Design review of the part built by this model. Coordinates are the model's own, in mm. Face numbers are marked on the shaded views. A direction names the side the tool comes from. Coordinates: 2 decimals unless noted, no trailing zeros. Write each loop counter-clockwise with the first axis right and the second up, starting at its lowest first coordinate (ties: lowest second). Pieces come first, ordered by that corner, then holes.
Q1. Add section C-C, the plane z = -10. Give the boundary of the cut face in (x, y), plus the area to 3 significant figures.
Q2. Add section B-B, the plane x = 0. Give the boundary of the cut face in (y, z), plus the area to 3 significant figures.
Q3. To check wall thickness, follow probe 1 along X at (y, z) = (1.05, 0); probe 2 along X at (y, z) = (-1, -18.5); probe 3 along Z at (x, y) = (0.25, -2). State the ranges of each line that lie inside material, in increasing order.
Q4. Add section D-D, the plane y = -1.25. Give the boundary of the cut face in (x, z), plus the area to 3 significant figures.
Q5. Add section A-A, the plane z = 0. Give the boundary of the cut face in (x, y), plus the area to 3 significant figures.
Q6. Clearance check with flat-ended pins moving along their axes: pin 1 Ø2 at (x, y) = (-3, 3.5) entering from +Z; pin 2 Ø2.5 at (x, y) = (-0.5, -2.5) entering from -Z; pin 3 Ø6 at (x, y) = (3.5, 7) entering from -Z. State where each tip first meets the part, or that it passes through.
Q7. Machinability: for the marked faces 1, 2, 3 and 4, which of the approach directions +Z, -Z, +X, -X, +Y, -Y give a long, thin tool a straight path to every point of the face, cutting with its end or side? Answer none if there is none.
from build123d import *

# Parameters (mm, degrees)
SKETCH_1_W      = 10
SKETCH_1_H      = 27
SKETCH_1_R      = 1.5
EXTRUDE_1_DEPTH = 1.6
SKETCH_2_W      = 8
SKETCH_2_H      = 2.5
EXTRUDE_2_DEPTH = 8
SKETCH_3_W      = 5
SKETCH_3_H      = 10
EXTRUDE_3_DEPTH = 6


with BuildPart() as part:
    # 草图1 → 凸台-拉伸1 (new body)
    with BuildSketch(Plane(origin=(0, 0, 0), x_dir=(1, 0, 0), z_dir=(0, 1, 0))):
        with Locations((0, 6.5)):
            Rectangle(SKETCH_1_W, SKETCH_1_H)
        with Locations(Location((0, 0, 0), (0, 0, 270))):
            Circle(SKETCH_1_R, mode=Mode.SUBTRACT)
    extrude(amount=EXTRUDE_1_DEPTH)

    # 草图2 → 凸台-拉伸2 (add)
    with BuildSketch(Plane(origin=(0, 1.6, 0), x_dir=(1, 0, 0), z_dir=(0, 1, 0))):
        with Locations((0, -5.25)):
            Rectangle(SKETCH_2_W, SKETCH_2_H)
    extrude(amount=EXTRUDE_2_DEPTH)

    # 草图3 → 凸台-拉伸3 (add)
    with BuildSketch(Plane.XZ):
        with Locations((0, -14.5)):
            Rectangle(SKETCH_3_W, SKETCH_3_H)
    extrude(amount=EXTRUDE_3_DEPTH)


solid = part.part
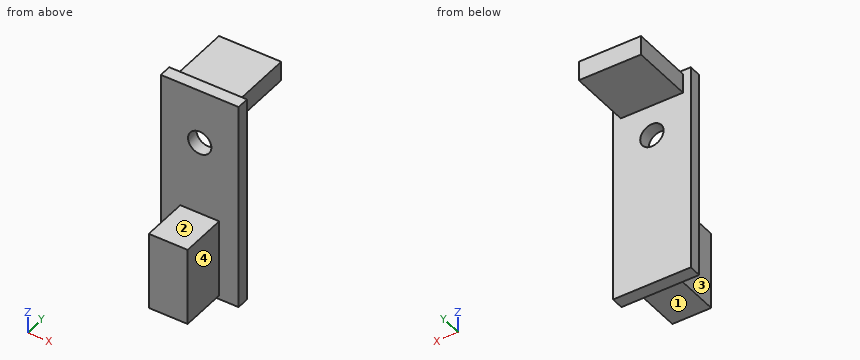
Here are the results:
1. outline: (-5, 0) - (-2.5, 0) - (-2.5, -6) - (2.5, -6) - (2.5, 0) - (5, 0) - (5, 1.6) - (-5, 1.6) - close
1. area: 46.0 mm2
2. outline: (-6, -19.5) - (0, -19.5) - (0, -20) - (1.6, -20) - (1.6, -1.5) - (0, -1.5) - (0, -9.5) - (-6, -9.5) - close; (0, 1.5) - (1.6, 1.5) - (1.6, 4) - (9.6, 4) - (9.6, 6.5) - (1.6, 6.5) - (1.6, 7) - (0, 7) - close
2. area: 118 mm2
3. probe 1: x = -5 to -1.5, 1.5 to 5
3. probe 2: x = -2.5 to 2.5
3. probe 3: z = -19.5 to -9.5
4. outline: (-2.5, -19.5) - (2.5, -19.5) - (2.5, -9.5) - (-2.5, -9.5) - close
4. area: 50.0 mm2
5. outline: (-5, 0) - (-1.5, 0) - (-1.5, 1.6) - (-5, 1.6) - close; (1.5, 0) - (5, 0) - (5, 1.6) - (1.5, 1.6) - close
5. area: 11.2 mm2
6. pin 1: stops at z = 6.5
6. pin 2: stops at z = -19.5
6. pin 3: stops at z = 4
7. face 1: -Z, +X, -X, -Y
7. face 2: +Z, +X, -X, -Y
7. face 3: +Z, -Z, -X, -Y
7. face 4: +Z, -Z, +X, -Y
